Autodesk Inventor part; units mm, degrees
ref_plane "YZ Plane" through (0, 0, 0) normal (1, 0, 0) x (0, 1, 0)
ref_plane "XZ Plane" through (0, 0, 0) normal (0, 1, 0) x (-1, 0, 0)
ref_plane "XY Plane" through (0, 0, 0) normal (0, 0, 1) x (1, 0, 0)
sketch "Sketch1" plane through (0, 0, 0) normal (0, 1, 0) x (-1, 0, 0)
  circle A0 centre (0, 0) radius 9.271
  dimension "d0" = 18.542
extrude "Extrusion1" add sketch "Sketch1" along normal blind 50.8
sketch "Sketch2" plane through (0, 50.8, 0) normal (0, 1, 0) x (1, 0, 0)
  line L0 (-2.54, 1.397) -> (2.54, 1.397)
  line L1 (2.54, 1.397) -> (2.54, -1.397)
  line L2 (2.54, -1.397) -> (-2.54, -1.397)
  line L3 (-2.54, -1.397) -> (-2.54, 1.397)
  line L4 (-2.54, 1.397) -> (2.54, -1.397) construction
  line L5 (2.54, 1.397) -> (-2.54, -1.397) construction
  point P0 (0, 0)
  point P1 (2.54, 0)
  point P2 (-2.54, 0)
  dimension "d3" = 2.794
  dimension "d4" = 5.08
extrude "Extrusion2" cut sketch "Sketch2" against normal blind 12.7
fillet "Fillet2" radius 0.635 2 edges at (9.271, 50.8, 0) (9.271, 0, 0)
sketch "Sketch3" plane through (2.54, 38.1, 1.397) normal (0, 0, -1) x (-1, 0, 0)
  line L0 (9.652, -0.635) -> (-4.572, -0.635)
  line L1 (-4.572, -0.635) -> (-4.572, -14.859)
  line L2 (-4.572, -14.859) -> (9.652, -14.859)
  line L3 (9.652, -14.859) -> (9.652, -0.635)
  line L4 (9.652, -0.635) -> (-4.572, -14.859) construction
  line L5 (-4.572, -0.635) -> (9.652, -14.859) construction
  line L6 (11.811, 12.065) -> (-6.731, 12.065)
  point P0 (2.54, -38.1)
  point P1 (2.54, -7.747)
  dimension "d9" = 14.224
  dimension "d10" = 14.224
  dimension "d11" = 12.7
extrude "Extrusion3" add sketch "Sketch3" along normal blind 127
sketch "Sketch4" plane through (2.54, 38.1, -125.603) normal (0, 0, -1) x (-1, 0, 0)
  line L0 (9.652, -0.635) -> (-4.572, -0.635)
  line L1 (-4.572, -14.859) -> (9.652, -14.859)
  line L2 (9.652, -0.635) -> (-4.572, -0.635)
  line L3 (-4.572, -0.635) -> (-4.572, -14.859)
  line L4 (-4.572, -14.859) -> (9.652, -14.859)
  line L5 (9.652, -14.859) -> (9.652, -0.635)
  point P0 (2.54, -38.1)
  point P1 (-4.572, -0.635)
extrude "Extrusion4" cut sketch "Sketch4" against normal blind 127
sketch "Sketch5" plane through (0, 50.8, 0) normal (0, 1, 0) x (1, 0, 0)
  circle A0 centre (0, 0) radius 2.54
  dimension "d16" = 5.08
extrude "Extrusion5" cut sketch "Sketch5" against normal blind 0.508
sketch "Sketch6" plane through (0, 50.8, 0) normal (0, 1, 0) x (1, 0, 0)
  arc A0 (-2.1213, -1.397) -> (2.1213, -1.397) centre (0, 0) ccw
  circle A1 centre (0, 0) radius 4.572
  dimension "d19" = 9.144
extrude "Extrusion6" cut sketch "Sketch6" against normal blind 0.254
properties part number "spinny"
Verification items for the finished model (mm, model axes). A direction names the side the tool comes from. Coordinates: 2 decimals unless noted, no trailing zeros. Write each loop counter-clockwise with the first axis right and the second up, starting at its lowest first coordinate (ties: lowest second). Pieces come first, ordered by that corner, then holes. Notation, with made-up numbers: (68, 47) - (123, 47) arc R35 cw to (123, 83) - close; hole circle Ø10 at (-31, 85). An arc over 180 degrees is marked (long way). Write item = value, one per line.
Q1. Access from +Z, -Z, +X, -X, +Y, -Y to the whole of each face (thin tool, end or side, straight path). Record for faces 5 (the face through (0, 37.465, -4)), 6 (the face through (0, 50.292, -2)), 7 (the face through (2.01, 25.05, 9.05)).
Answer:
face_5 = -Z
face_6 = +Y
face_7 = +Y, -Y
Q2. Material ranges on L1, parallel to Y at x = 6.75, z = -3.25 (3 decimals); L2, parallel to Y at x = -2.75, z = 3; L3, parallel to Z at x = 0, y = 50.7, recorded low to high. Write a range as from..to.
Answer:
L1 = 0..23.241, 37.465..50.8
L2 = 0..50.55
L3 = -8.98..-4.57, 4.57..8.98
Q3. Mould release check, pull along Y, two halves, no side actions. Record for faces 1 (the face through (-4, 50.8, -4)), 2 (the face through (0, 0, 0)), 3 (the face through (0, 44, -1.397)), 4 (the face through (7.112, 30, -2)): released by +Y, released by -Y, zero draft, split by the parting line, or undercut.
Answer:
face_1 = released by +Y
face_2 = released by -Y
face_3 = zero draft
face_4 = undercut
Q4. Cross-section at C-C (y = 36). Enter the section's corners in (x, z).
Answer:
outline = (-7.11, -5.95) - (-7.11, 1.4) - (7.11, 1.4) - (7.11, -5.95) arc R9.27 ccw (long way) to start
Q5. Cross-section at B-B (x = 0). Enter the section's corners in (y, z) (3 decimals), plus the area to 3 significant figures.
Answer:
outline = (0, -8.636) arc R0.635 ccw to (0.635, -9.271) - (23.241, -9.271) - (23.241, 1.397) - (37.465, 1.397) - (37.465, -9.271) - (50.165, -9.271) arc R0.635 ccw to (50.8, -8.636) - (50.8, -4.572) - (50.546, -4.572) - (50.546, -2.54) - (50.292, -2.54) - (50.292, -1.397) - (38.1, -1.397) - (38.1, 1.397) - (50.292, 1.397) - (50.292, 2.54) - (50.546, 2.54) - (50.546, 4.572) - (50.8, 4.572) - (50.8, 8.636) arc R0.635 ccw to (50.165, 9.271) - (0.635, 9.271) arc R0.635 ccw to (0, 8.636) - close
area = 752 mm²
Q6. Go/stop test with flat-tipped pins: pin 1 Ø1.5 at (y, z) = (38, -6) entering from +X; pin 2 Ø6 at (x, y) = (-5.5, 24) entering from +Z; pin 3 Ø0.9 at (x, z) = (0, 2) entering from +Y. Record where each tip stops, or that it passes through.
Answer:
pin_1 = 7.64
pin_2 = 8.93
pin_3 = 50.29
Q7. Cross-section at A-A (z = 0). Enter the section's corners in (x, y) (3 decimals).
Answer:
outline = (-9.271, 0.635) arc R0.635 ccw to (-8.636, 0) - (8.636, 0) arc R0.635 ccw to (9.271, 0.635) - (9.271, 50.165) arc R0.635 ccw to (8.636, 50.8) - (4.572, 50.8) - (4.572, 50.546) - (2.54, 50.546) - (2.54, 38.1) - (-2.54, 38.1) - (-2.54, 50.546) - (-4.572, 50.546) - (-4.572, 50.8) - (-8.636, 50.8) arc R0.635 ccw to (-9.271, 50.165) - close; hole (-7.112, 23.241) - (7.112, 23.241) - (7.112, 37.465) - (-7.112, 37.465) - close
